Answer from the drawing. Dimensions are ordinates in mm from the lowest x, y and z of the part. A direction names the side the tool comes from. Round coordinates to 2 decimals unless told otherwise and drop trailing zeros. Loops run counter-clockwise (first coordinate to the right, second up) from the corner with the lowest first, then second, coordinate; pieces in that order, holes last. Notation, with made-up numbers: (-31.5, 65.5) -> (-13.5, 65.5) arc R20 ccw to (-13.5, 94.5) -> close; hole circle Ø9 at (74, 77.5). An arc over 180 degrees is marked (long way). One line per question, with ' | ' between items.
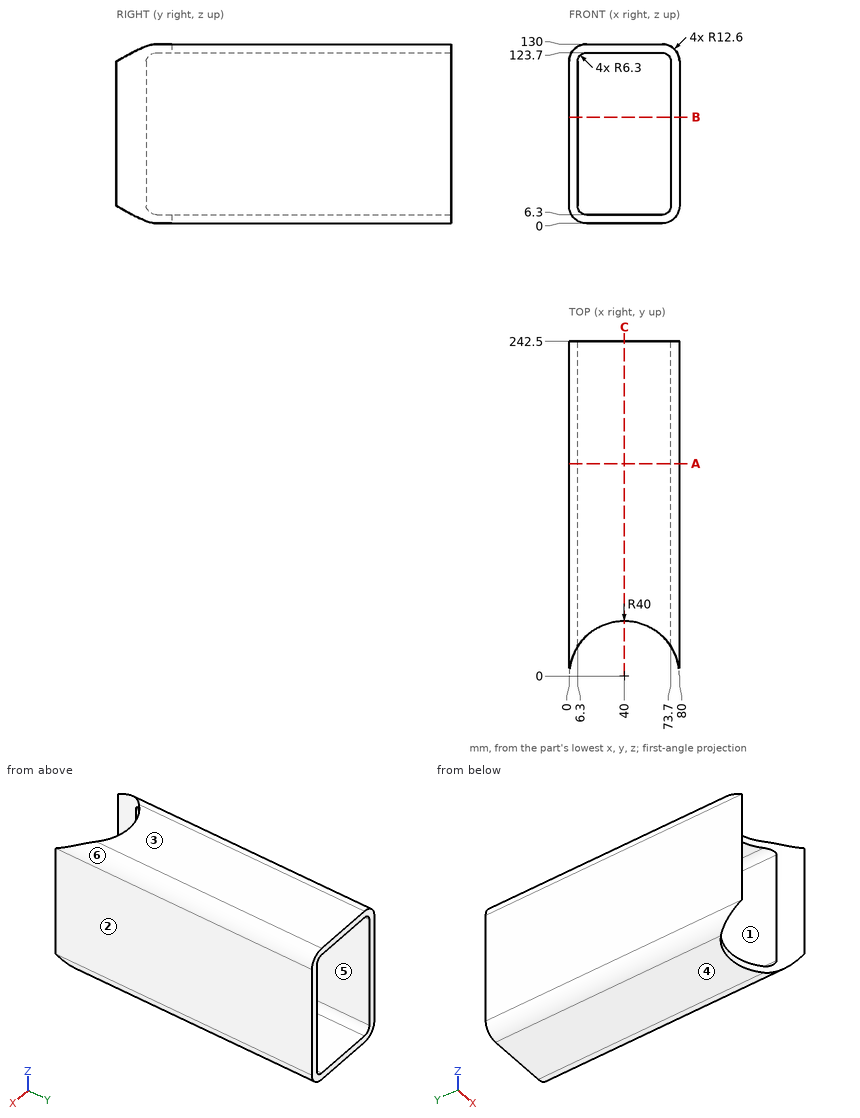
Q1. For a pull along Z with two mould halves and no side action, classify the marked faces 1, 2, 3 and 4 as pulls with the +Z half, pulls with the -Z half, needs draft (parallel to the pull), parting line crosses it, or undercut.
Numbers:
face 1: undercut | face 2: needs draft | face 3: pulls with the +Z half | face 4: pulls with the -Z half
Q2. For the marked faces 5 and 6, determine the directions among +Z, -Z, +X, -X, +Y, -Y from which every point of the face is accessible in a straight line to the end or side of a thin tool.
Numbers:
face 5: +Y, -Y | face 6: +Z, +X, +Y, -Y
Q3. A cutting plane is placed at C-C on x = 40. Give the vertices of the cut face in (y, z).
Numbers:
outline: (40, 0) -> (242.5, 0) -> (242.5, 6.3) -> (40, 6.3) -> close; (40, 123.7) -> (242.5, 123.7) -> (242.5, 130) -> (40, 130) -> close
Q4. Find the intervals of material crossed by line 1 (X direction, y = 197, z = 43); line 2 (Z direction, x = 39.5, y = 94); line 3 (X direction, y = 18, z = 29), in increasing order. Write a range as from..to.
Numbers:
line 1: 0..6.3, 73.7..80 | line 2: 0..6.3, 123.7..130 | line 3: 0..4.28, 75.72..80
Q5. A cutting plane is placed at B-B on z = 77. Give the vertices of the cut face in (x, y), plus the area to 3 significant figures.
Numbers:
outline: (0, 0) arc R40 cw to (6.3, 21.55) -> (6.3, 242.5) -> (0, 242.5) -> close; (73.7, 21.55) arc R40 cw to (80, 0) -> (80, 242.5) -> (73.7, 242.5) -> close | area: 2,870 mm^2
Q6. A cutting plane is placed at A-A on y = 154. Give the vertices of the cut face in (x, z), plus the area to 3 significant figures.
Numbers:
outline: (0, 12.6) arc R12.6 ccw to (12.6, 0) -> (67.4, 0) arc R12.6 ccw to (80, 12.6) -> (80, 117.4) arc R12.6 ccw to (67.4, 130) -> (12.6, 130) arc R12.6 ccw to (0, 117.4) -> close; hole (6.3, 12.6) arc R6.3 ccw to (12.6, 6.3) -> (67.4, 6.3) arc R6.3 ccw to (73.7, 12.6) -> (73.7, 117.4) arc R6.3 ccw to (67.4, 123.7) -> (12.6, 123.7) arc R6.3 ccw to (6.3, 117.4) -> close | area: 2,390 mm^2
